from build123d import *

# Parameters (mm, degrees)
CYLINDER_R     = 5.2
CYLINDER_DEPTH = 132


with BuildPart() as cono:
    # Cone → Cone (revolve)
    with BuildSketch(Plane(origin=(0, 0, -12), x_dir=(1, 0, 0), z_dir=(0, -1, 0))):
        Polygon((0, 0), (5.2, 12), (0, 12), align=None)
    revolve(axis=Axis((0, 0, -12), (0, 0, 1)))


with BuildPart() as obj1:
    # Cylinder → Cylinder (new body)
    with BuildSketch(Plane.XY):
        Circle(CYLINDER_R)
    extrude(amount=CYLINDER_DEPTH)

    # Fusion004: union Cono
    add(cono.part)


with BuildPart() as obj1_1:
    # Fusion004 placement: moved
    add(obj1.part.moved(Location((0, 0, -24))))


solid = obj1_1.part
For this review, take the finished solid that the model builds, in its own axes (mm). Round coordinates to 2 decimals unless told otherwise and drop trailing zeros. Loops run counter-clockwise (first coordinate to the right, second up) from the corner with the lowest first, then second, coordinate; pieces in that order, holes last. Notation, with made-up numbers: (59, 42) - (98, 42) arc R37 cw to (98, 78) - close; hole circle Ø10 at (-24, 70.25). An arc over 180 degrees is marked (long way). One line per item, written item: value. Start each with the question number.
Item 1: Take a section at A-A (z = 16). Give the boundary of the cut face in (x, y), plus the area to 3 significant figures.
Item 2: For L1, parallel to Y at x = 2.75, z = 79.5; L2, parallel to X at y = 2.5, z = 101.5, list the stretches that pass through material, from the lowest coordinate up.
Item 3: Clearance check with flat-ended pins moving along their axes: pin 1 Ø2 at (x, z) = (3.5, 43.5) entering from +Y; pin 2 Ø1.5 at (y, z) = (-2, 74) entering from -X. State where each tip first meets the part, or that it passes through.
Answer below:
1. outline: circle Ø10.4 at (0, 0)
1. area: 84.9 mm2
2. L1: y = -4.41 to 4.41
2. L2: x = -4.56 to 4.56
3. pin 1: stops at y = 4.56
3. pin 2: stops at x = -5.05
